Verification items for the finished model (mm, model axes). A direction names the side the tool comes from. Give positions to 0.01 mm unless a question says otherwise; leave off trailing zeros. Loops run counter-clockwise (first coordinate to the right, second up) from the corner with the lowest first, then second, coordinate; pieces in that order, holes last. Notation, with made-up numbers: (75, 82) - (124, 82) arc R25 ccw to (124, 110) - close; hole circle Ø6 at (-25, 45.5). An arc over 180 degrees is marked (long way). Use one line per item in the form item = value.
```python
from build123d import *

# Parameters (mm, degrees)
F0_W     = 10
F0_H     = 20
F1_DEPTH = 5
F3_DEPTH = 30
F5_DEPTH = 80


with BuildPart() as f1:
    # F0 (on Top) → F1 (new body)
    with BuildSketch(Plane.XY):
        with BuildLine():
            Line((150, -25), (100, -25))
            ThreePointArc((100, -25), (64.644661, -10.355339), (50, 25))
            Line((50, 25), (0, 25))
            Line((0, 25), (0, -55))
            Line((0, -55), (150, -55))
            Line((150, -55), (150, -25))
        make_face()
        with Locations((15, 10)):
            Rectangle(F0_W, F0_H, mode=Mode.SUBTRACT)
    extrude(amount=F1_DEPTH)

    # F2 (on face) → F3 (join)
    with BuildSketch(Plane.XY.offset(5)):
        Polygon((30, 25), (0, 25), (0, -55), (2, -55), (2, 23), (28, 23), (28, -55), (30, -55), align=None)
    extrude(amount=F3_DEPTH)

    # F4 (on face) → F5 (join, through all)
    with BuildSketch(Plane(origin=(0, 25, 0), x_dir=(-1, 0, 0), z_dir=(0, 1, 0))):
        Polygon((-15, 60.980762), (-30, 35), (0, 35), align=None)
    extrude(amount=-F5_DEPTH)


solid = f1.part
```
1. Tool access check on faces 5 (the flat face through (0, -14, 17)), 6 (the flat face through (125, -25, 2)), 7 (the flat face through (10, 10, 2)), 8 (the flat face through (30, -16, 20)), 9 (the flat face through (28, -15, 20)). Record the directions out of +Z, -Z, +X, -X, +Y, -Y that give a thin tool (end or side, any length) a straight path to the whole face; none if there is none.
Result set:
face_5 = +Z, -Z, -X, +Y, -Y
face_6 = +Z, -Z, +X, +Y
face_7 = -Z
face_8 = +Z, +X, +Y, -Y
face_9 = -Y
2. Section check D-D, the plane x = 25.5. Record the cut outline in (y, z), then the cut area to 3 significant figures.
Result set:
outline = (-55, 0) - (25, 0) - (25, 42.79) - (-55, 42.79) - (-55, 35) - (23, 35) - (23, 5) - (-55, 5) - close
area = 1,080 mm²
3. Depth check by flat-ended pin: pin 1 Ø2 at (y, z) = (-13.5, 10.5) entering from -X; pin 2 Ø5.5 at (x, z) = (125, 3.5) entering from +Y; pin 3 Ø8 at (y, z) = (4, 48.5) entering from -X; pin 4 Ø10 at (x, y) = (127, -40.5) entering from +Z. Enter the tip coordinate at first touch or a pass-through.
Result set:
pin_1 = 0
pin_2 = -25
pin_3 = 5.48
pin_4 = 5
4. Draft check along Z on faces 1 (the flat face through (2, -17, 20)), 2 (the flat face through (15, -15, 5)), 3 (the flat face through (15, 0, 2)), 4 (the flat face through (7.395, -14.44, 47.809)). Enter one of: released by +Z, released by -Z, zero draft, split by the parting line, or undercut.
Result set:
face_1 = undercut
face_2 = undercut
face_3 = zero draft
face_4 = released by +Z
5. Section check B-B, the plane y = 5. Record the cut outline in (x, z), then the cut area to 3 significant figures.
Result set:
outline = (0, 0) - (10, 0) - (10, 5) - (2, 5) - (2, 35) - (28, 35) - (28, 5) - (20, 5) - (20, 0) - (54.17, 0) - (54.17, 5) - (30, 5) - (30, 35) - (15, 60.98) - (0, 35) - close
area = 731 mm²
6. Section check A-A, the plane z = 19.5. Record the cut outline in (x, y), then the cut area to 3 significant figures.
Result set:
outline = (0, -55) - (2, -55) - (2, 23) - (28, 23) - (28, -55) - (30, -55) - (30, 25) - (0, 25) - close
area = 372 mm²
7. Section check C-C, the plane x = 44. Record the cut outline in (y, z), then the cut area to 3 significant figures.
Result set:
outline = (-55, 0) - (25, 0) - (25, 5) - (-55, 5) - close
area = 400 mm²
8. Scan lines: probe 1 along X at (y, z) = (2.5, 21.5); probe 2 along Z at (x, y) = (68.5, -17.5); probe 3 along Y at (x, z) = (24, 5.5). Record each from-to range of solid material in increasing order.
Result set:
probe_1 = 0 to 2, 28 to 30
probe_2 = 0 to 5
probe_3 = 23 to 25
